Here's how the part is built. I have some questions about the finished solid (model axes, mm). Face numbers are marked on the shaded views. A direction names the side the tool comes from. Coordinates: 2 decimals unless noted, no trailing zeros. Order: outer loops, then holes, each group sorted by start corner. A loop starts at its lowest first (then second) coordinate and runs counter-clockwise, first axis right, second up.
```python
from build123d import *

# Parameters (mm, degrees)
F0_R     = 20
F0_R_2   = 9.5
F1_DEPTH = 1
F6_DEPTH = 5
F7_COUNT = 9
F8_R     = 1
F9_DEPTH = 5


with BuildPart() as f1:
    # F0 (on Top) → F1 (new body)
    with BuildSketch(Plane.XY):
        Circle(F0_R)
        Circle(F0_R_2, mode=Mode.SUBTRACT)
        Circle(F0_R_2)
    extrude(amount=F1_DEPTH)

    # F5 (on line) → F6 (join, symmetric)
    with BuildSketch(Plane(origin=(-12.5, 0, 0), x_dir=(0, -1, 0), z_dir=(-1, 0, 0))):
        Polygon((2.0567882708, 0), (-2.0567882708, 0), (0, -2.5773376692), align=None)
    extrude(amount=F6_DEPTH, both=True)

    # F7: F1 ×9 about axis
    f7_axis = Axis((0, 0, 0), (0, 0, 1))


with BuildPart() as f1_1:
    add(f1.part)
    for i in range(1, F7_COUNT):
        add(f1.part.rotate(f7_axis, i * 360 / F7_COUNT))

    # F8
    f8_edges = [f1_1.edges().sort_by_distance(p)[0] for p in [
        (-12.5, 0, -2.577338),
        (-9.575556, 8.034845, -2.577338),
        (-2.170602, 12.310097, -2.577338),
        (6.25, 10.825318, -2.577338),
        (11.746158, 4.275252, -2.577338),
        (11.746158, -4.275252, -2.577338),
        (6.25, -10.825318, -2.577338),
        (-2.170602, -12.310097, -2.577338),
        (-9.575556, -8.034845, -2.577338),
    ]]
    fillet(f8_edges, radius=F8_R)

    # F0 (on Top) → F9 (cut, symmetric)
    with BuildSketch(Plane.XY):
        Circle(F0_R_2)
    extrude(amount=F9_DEPTH, both=True, mode=Mode.SUBTRACT)


solid = f1_1.part
```
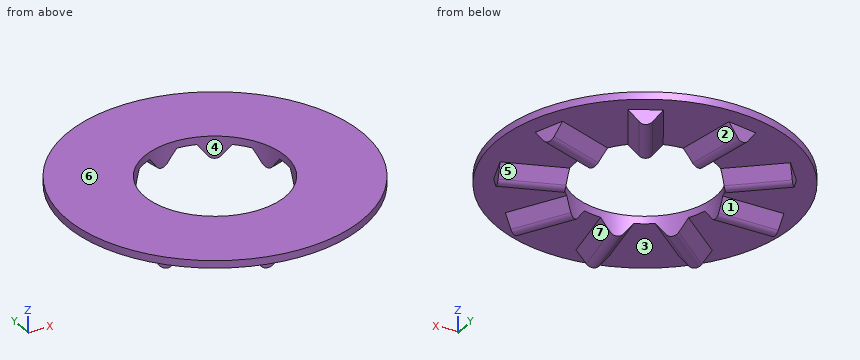
Q1. I need wall thicknesses on L1, parallel to Y at x = 0, z = 0.15; L2, parallel to X at y = -11.5, z = -1.55. Which ranges of each line are inside material? Lowest first, please.
Q2. Will these pins go through, and if not, where does the flat tip stop? pin 1 (1 mm diameter, centred on x = -6, y = 10, fed in from -Z); pin 2 (1 mm diameter, centred on y = -1, z = -1, fed in from -X); pin 3 (17 mm diameter, centred on x = 0, y = 0, fed in from -Z).
Q3. For the marked faces 1, 2, 3 and 4, which set-ups out of +Z, -Z, +X, -X, +Y, -Y let a thin tool reach every point of the face, with its end or its side?
Q4. If we section it at A-A on x = -17: Write out the boundary of the cut face in (y, z), then the cut area to 3 significant figures.
Q5. We'd pull the mould along X, two halves only. Please class the marked faces 5, 6 and 7: pulls with the +X half, pulls with the -X half, needs draft (parallel to the pull), parting line crosses it, or undercut.
Reply:
1. L1: y = -20 to -9.5, 9.5 to 20
1. L2: x = -13.19 to -12.43, -2.86 to -1.2, 5.69 to 7.59
2. pin 1: stops at z = 0
2. pin 2: stops at x = -17.5
2. pin 3: passes through
3. face 1: -Z, -X
3. face 2: -Z, +Y
3. face 3: -Z
3. face 4: +Z, -Z
4. outline: (-10.54, 0) - (-2.06, 0) - (-0.78, -1.6) arc R1 ccw to (0.78, -1.6) - (2.06, 0) - (10.54, 0) - (10.54, 1) - (-10.54, 1) - close
4. area: 26.0 mm2
5. face 5: pulls with the +X half
5. face 6: needs draft
5. face 7: undercut
